Drawing for the job (mm, zero at the part's lowest x, y, z). A direction names the side the tool comes from. Coordinates: 2 decimals unless noted, no trailing zeros. Write each loop counter-clockwise with the first axis right and the second up, starting at its lowest first coordinate (ties: lowest second). Pieces come first, ordered by that corner, then holes. Notation, with made-up numbers: (-7.75, 13.5) -> (14.25, 13.5) arc R19 ccw to (14.25, 34.5) -> close; hole circle Ø5 at (58, 29). An arc over 180 degrees is marked (long way). Answer as CSV lines item,"result". Start each with the question number.
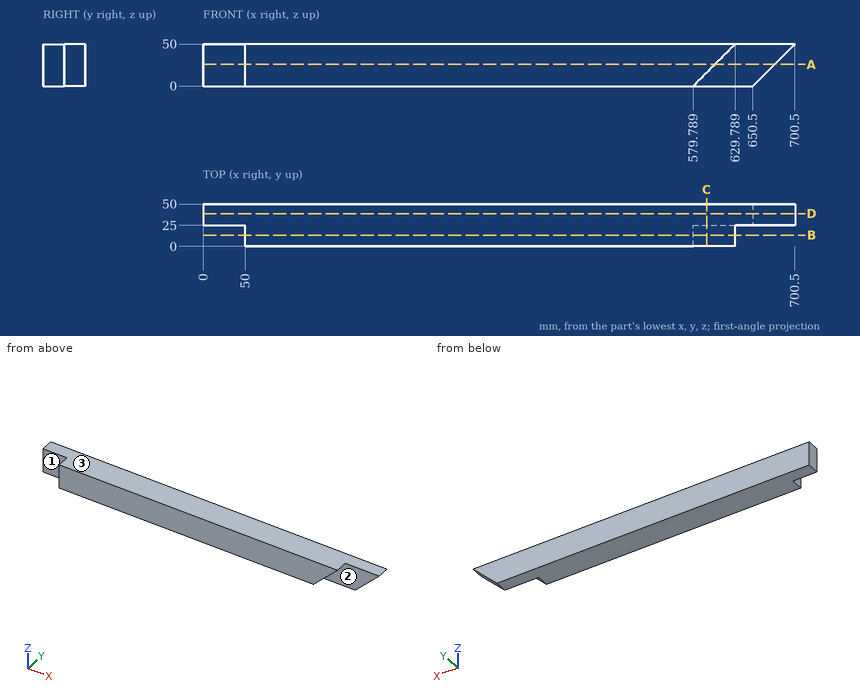
1. Tool access for the marked faces 1, 2 and 3: list every direction of +Z, -Z, +X, -X, +Y, -Y with a clear straight run to the whole face (end or side of a thin tool).
2. Cut at C-C (x = 596). Give the cut face in (y, z), then the cut area to 3 significant figures.
3. Flat gauge pins, fed straight in: P1, Ø25, axis at x = 29.5, z = 24, coming from the -Y side; P2, Ø20, axis at y = 12, z = 25, coming from the -X side. Where does each tip first touch, or does it go through?
4. Cut at B-B (y = 13.5). Give the cut face in (x, z), then the cut area to 3 significant figures.
5. Cut at D-D (y = 39). Give the cut face in (x, z), then the cut area to 3 significant figures.
6. Cut at A-A (z = 26). Give the cut face in (x, y).
7. Wall check: line 1 (Y direction, x = 657, z = 27.5); line 2 (X direction, y = 48, z = 24.5); line 3 (X direction, y = 10, z = 35). Give the ranges that are in metal, low to high.
Geometry check:
1,face 1,"+Z, -Z, -X, -Y"
1,face 2,"-Z, +X, -Y"
1,face 3,"+Z, +X, -X, +Y, -Y"
2,outline,"(0, 16.21) -> (25, 16.21) -> (25, 0) -> (50, 0) -> (50, 50) -> (0, 50) -> close"
2,area,"2,090 mm²"
3,P1,"y = 25"
3,P2,"x = 50"
4,outline,"(50, 0) -> (579.79, 0) -> (629.79, 50) -> (50, 50) -> close"
4,area,"27,700 mm²"
5,outline,"(0, 0) -> (650.5, 0) -> (700.5, 50) -> (0, 50) -> close"
5,area,"33,800 mm²"
6,outline,"(0, 25) -> (50, 25) -> (50, 0) -> (605.79, 0) -> (605.79, 25) -> (676.5, 25) -> (676.5, 50) -> (0, 50) -> close"
7,line 1,"25 to 50"
7,line 2,"0 to 675"
7,line 3,"50 to 614.79"
